The model under review builds one solid part; all positions refer to its coordinate system, in mm. Face numbers are marked on the shaded views. Give positions to 0.01 mm unless a question says otherwise; leave off trailing zeros. Order: outer loops, then holes, each group sorted by start corner. A loop starts at its lowest first (then second) coordinate and runs counter-clockwise, first axis right, second up. Notation, with made-up numbers: (-5, -39.75) - (16, -39.75) arc R27 cw to (16, -17.75) - close; hole circle Ø6 at (74, -15). An arc over 180 degrees is marked (long way). Use CSV: the item, a comma, the result in double quotes. Start each with the question number.
1. To check wall thickness, follow line 1 (Z direction, x = -6, y = 1.75); line 2 (Y direction, x = -7.25, z = -5.5); line 3 (X direction, y = 0.3, z = -4). State the ranges of each line that lie inside material, in increasing order. Write a range as [from, to].
2. Draft analysis for pull direction Z (two halves, no side actions). For the marked faces 1, 2, 3 and 4, state which applies: released by +Z, released by -Z, zero draft, split by the parting line, or undercut.
3. Take a section at D-D, the plane x = 7. State the section outline as (y, z) points.
4. Take a section at A-A, the plane x = 5. State the section outline as (y, z) points, then the cut area to 3 significant figures.
5. For pin 1 (2 mm diameter, centred on y = 3.5, z = -2.5, fed in from -X); pin 2 (1.5 mm diameter, centred on x = 1, y = 1.5, fed in from -Z); pin 3 (1 mm diameter, centred on y = 1.5, z = 6.5, fed in from +X), all flat-tipped, find the tip position at first contact; note any pin that passes through.
6. Take a section at B-B, the plane y = 0.6. State the section outline as (x, z) points, then the cut area to 3 significant figures.
7. Take a section at C-C, the plane x = -7.5. State the section outline as (y, z) points, then the cut area to 3 significant figures.
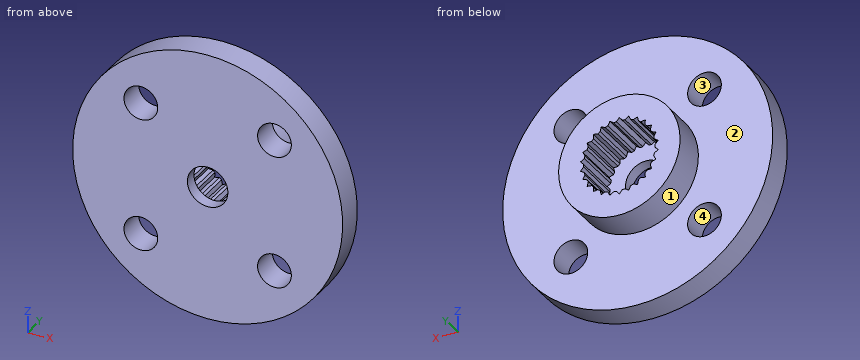
```python
from build123d import *

# Parameters (mm, degrees)
SKETCH_1_W              = 10
SKETCH_1_H              = 2
SKETCH_2_R              = 4.5
EXTRUDE_1_DEPTH         = 2.5
CUT_EXTRUDE_1_DEPTH     = 3.6
HOLE_WIZARD_3_0_3_1_D   = 3
HOLE_WIZARD_2_5_2_5_1_D = 2.5
CHAMFER_1_SIZE          = 0.140560122
CHAMFER_1_EDGE_2_SIZE   = 0.140560122
CHAMFER_1_EDGE_3_SIZE   = 0.140560122
CHAMFER_1_EDGE_4_SIZE   = 0.140560122
CHAMFER_1_EDGE_5_SIZE   = 0.140560122
CHAMFER_1_EDGE_6_SIZE   = 0.140560122
CHAMFER_1_EDGE_7_SIZE   = 0.140560122
CHAMFER_1_EDGE_8_SIZE   = 0.140560122
CHAMFER_1_EDGE_9_SIZE   = 0.140560122
CHAMFER_1_EDGE_10_SIZE  = 0.140560122
CHAMFER_1_EDGE_11_SIZE  = 0.140560122
CHAMFER_1_EDGE_12_SIZE  = 0.140560122
CHAMFER_1_EDGE_13_SIZE  = 0.140560122
CHAMFER_1_EDGE_14_SIZE  = 0.140560122
CHAMFER_1_EDGE_15_SIZE  = 0.140560122
CHAMFER_1_EDGE_16_SIZE  = 0.140560122
CHAMFER_1_EDGE_17_SIZE  = 0.140560122
CHAMFER_1_EDGE_18_SIZE  = 0.140560122
CHAMFER_1_EDGE_19_SIZE  = 0.140560122
CHAMFER_1_EDGE_20_SIZE  = 0.140560122
CHAMFER_1_EDGE_21_SIZE  = 0.140560122
CHAMFER_1_EDGE_22_SIZE  = 0.140560122
CHAMFER_1_EDGE_23_SIZE  = 0.140560122
CHAMFER_1_EDGE_24_SIZE  = 0.140560122
CHAMFER_1_EDGE_25_SIZE  = 0.140560122
CHAMFER_1_EDGE_26_SIZE  = 0.140560122


with BuildPart() as part:
    # Эскиз1 → Повернуть1 (revolve)
    with BuildSketch(Plane.XY, mode=Mode.PRIVATE) as revolve_1_sk:
        with Locations((5, 1)):
            Rectangle(SKETCH_1_W, SKETCH_1_H)
    revolve(revolve_1_sk.sketch.rotate(Axis((0, 2, 0), (0, -1, 0)), 270), axis=Axis((0, 2, 0), (0, -1, 0)))

    # Эскиз2 → Бобышка-Вытянуть1 (add)
    with BuildSketch(Plane(origin=(0, 2, 0), x_dir=(-1, 0, 0), z_dir=(0, 1, 0))):
        with Locations(Location((0, 0, 0), (0, 0, 90))):
            Circle(SKETCH_2_R)
    extrude(amount=EXTRUDE_1_DEPTH)

    # Эскиз3 → Вырез-Вытянуть1 (cut)
    with BuildSketch(Plane(origin=(0, 4.5, 0), x_dir=(-1, 0, 0), z_dir=(0, 1, 0))):
        Polygon((-2.711547104, 1.028354172), (-2.477853855, 0.610736123), (-2.878855735, 0.349556373), (-2.552010646, 0), (-2.878855735, -0.349556373), (-2.477853855, -0.610736123), (-2.711547104, -1.028354172), (-2.259693204, -1.185978483), (-2.386653211, -1.647387766), (-1.910207398, -1.692296084), (-1.923055709, -2.17068117), (-1.449707281, -2.100263587), (-1.347697199, -2.567822474), (-0.904955447, -2.386171406), (-0.694015426, -2.815731271), (-0.307610891, -2.533403615), (0, -2.9), (0.307610891, -2.533403615), (0.694015426, -2.815731271), (0.904955447, -2.386171406), (1.347697199, -2.567822474), (1.449707281, -2.100263587), (1.923055709, -2.17068117), (1.910207398, -1.692296084), (2.386653211, -1.647387766), (2.259693204, -1.185978483), (2.711547104, -1.028354172), (2.477853855, -0.610736123), (2.878855735, -0.349556373), (2.552010646, 0), (2.878855735, 0.349556373), (2.477853855, 0.610736123), (2.711547104, 1.028354172), (2.259693204, 1.185978483), (2.386653211, 1.647387766), (1.910207398, 1.692296084), (1.923055709, 2.17068117), (1.449707281, 2.100263587), (1.347697199, 2.567822474), (0.904955447, 2.386171406), (0.694015426, 2.815731271), (0.307610891, 2.533403615), (0, 2.9), (-0.307610891, 2.533403615), (-0.694015426, 2.815731271), (-0.904955447, 2.386171406), (-1.347697199, 2.567822474), (-1.449707281, 2.100263587), (-1.923055709, 2.17068117), (-1.910207398, 1.692296084), (-2.386653211, 1.647387766), (-2.259693204, 1.185978483), align=None)
    extrude(amount=-CUT_EXTRUDE_1_DEPTH, mode=Mode.SUBTRACT)

    # Диаметр отверстия Ø3.0 (3)1 (through all)
    with Locations(Plane(origin=(0, 0.9, 0), x_dir=(1, 0, 0), z_dir=(0, 1, 0))):
        with Locations((0, 0)):
            Hole(HOLE_WIZARD_3_0_3_1_D / 2)

    # Диаметр отверстия Ø2.5 (2.5)1 (through all)
    with Locations(Plane(origin=(0, 2, 0), x_dir=(1, 0, 0), z_dir=(0, 1, 0))):
        with Locations((-4.949747468, 4.949747468), (4.949747468, 4.949747468), (4.949747468, -4.949747468), (-4.949747468, -4.949747468)):
            Hole(HOLE_WIZARD_2_5_2_5_1_D / 2)

    # Фаска1
    chamfer_1_edges = [part.edges().sort_by_distance(p)[0] for p in [
        (2.259693204, 2.7, 1.185978483),
    ]]
    chamfer(chamfer_1_edges, length=CHAMFER_1_SIZE)

    # Фаска1 edge 2
    chamfer_1_edge_2_edges = [part.edges().sort_by_distance(p)[0] for p in [
        (1.910207398, 2.7, 1.692296084),
    ]]
    chamfer(chamfer_1_edge_2_edges, length=CHAMFER_1_EDGE_2_SIZE)

    # Фаска1 edge 3
    chamfer_1_edge_3_edges = [part.edges().sort_by_distance(p)[0] for p in [
        (1.449707281, 2.7, 2.100263587),
    ]]
    chamfer(chamfer_1_edge_3_edges, length=CHAMFER_1_EDGE_3_SIZE)

    # Фаска1 edge 4
    chamfer_1_edge_4_edges = [part.edges().sort_by_distance(p)[0] for p in [
        (0.904955447, 2.7, 2.386171406),
    ]]
    chamfer(chamfer_1_edge_4_edges, length=CHAMFER_1_EDGE_4_SIZE)

    # Фаска1 edge 5
    chamfer_1_edge_5_edges = [part.edges().sort_by_distance(p)[0] for p in [
        (0.307610891, 2.7, 2.533403615),
    ]]
    chamfer(chamfer_1_edge_5_edges, length=CHAMFER_1_EDGE_5_SIZE)

    # Фаска1 edge 6
    chamfer_1_edge_6_edges = [part.edges().sort_by_distance(p)[0] for p in [
        (-0.307610891, 2.7, 2.533403615),
    ]]
    chamfer(chamfer_1_edge_6_edges, length=CHAMFER_1_EDGE_6_SIZE)

    # Фаска1 edge 7
    chamfer_1_edge_7_edges = [part.edges().sort_by_distance(p)[0] for p in [
        (-0.904955447, 2.7, 2.386171406),
    ]]
    chamfer(chamfer_1_edge_7_edges, length=CHAMFER_1_EDGE_7_SIZE)

    # Фаска1 edge 8
    chamfer_1_edge_8_edges = [part.edges().sort_by_distance(p)[0] for p in [
        (-1.449707281, 2.7, 2.100263587),
    ]]
    chamfer(chamfer_1_edge_8_edges, length=CHAMFER_1_EDGE_8_SIZE)

    # Фаска1 edge 9
    chamfer_1_edge_9_edges = [part.edges().sort_by_distance(p)[0] for p in [
        (-1.910207398, 2.7, 1.692296084),
    ]]
    chamfer(chamfer_1_edge_9_edges, length=CHAMFER_1_EDGE_9_SIZE)

    # Фаска1 edge 10
    chamfer_1_edge_10_edges = [part.edges().sort_by_distance(p)[0] for p in [
        (-2.259693204, 2.7, 1.185978483),
    ]]
    chamfer(chamfer_1_edge_10_edges, length=CHAMFER_1_EDGE_10_SIZE)

    # Фаска1 edge 11
    chamfer_1_edge_11_edges = [part.edges().sort_by_distance(p)[0] for p in [
        (-2.477853855, 2.7, 0.610736123),
    ]]
    chamfer(chamfer_1_edge_11_edges, length=CHAMFER_1_EDGE_11_SIZE)

    # Фаска1 edge 12
    chamfer_1_edge_12_edges = [part.edges().sort_by_distance(p)[0] for p in [
        (-2.552010646, 2.7, 0),
    ]]
    chamfer(chamfer_1_edge_12_edges, length=CHAMFER_1_EDGE_12_SIZE)

    # Фаска1 edge 13
    chamfer_1_edge_13_edges = [part.edges().sort_by_distance(p)[0] for p in [
        (-2.477853855, 2.7, -0.610736123),
    ]]
    chamfer(chamfer_1_edge_13_edges, length=CHAMFER_1_EDGE_13_SIZE)

    # Фаска1 edge 14
    chamfer_1_edge_14_edges = [part.edges().sort_by_distance(p)[0] for p in [
        (-2.259693204, 2.7, -1.185978483),
    ]]
    chamfer(chamfer_1_edge_14_edges, length=CHAMFER_1_EDGE_14_SIZE)

    # Фаска1 edge 15
    chamfer_1_edge_15_edges = [part.edges().sort_by_distance(p)[0] for p in [
        (-1.910207398, 2.7, -1.692296084),
    ]]
    chamfer(chamfer_1_edge_15_edges, length=CHAMFER_1_EDGE_15_SIZE)

    # Фаска1 edge 16
    chamfer_1_edge_16_edges = [part.edges().sort_by_distance(p)[0] for p in [
        (-1.449707281, 2.7, -2.100263587),
    ]]
    chamfer(chamfer_1_edge_16_edges, length=CHAMFER_1_EDGE_16_SIZE)

    # Фаска1 edge 17
    chamfer_1_edge_17_edges = [part.edges().sort_by_distance(p)[0] for p in [
        (-0.904955447, 2.7, -2.386171406),
    ]]
    chamfer(chamfer_1_edge_17_edges, length=CHAMFER_1_EDGE_17_SIZE)

    # Фаска1 edge 18
    chamfer_1_edge_18_edges = [part.edges().sort_by_distance(p)[0] for p in [
        (-0.307610891, 2.7, -2.533403615),
    ]]
    chamfer(chamfer_1_edge_18_edges, length=CHAMFER_1_EDGE_18_SIZE)

    # Фаска1 edge 19
    chamfer_1_edge_19_edges = [part.edges().sort_by_distance(p)[0] for p in [
        (0.307610891, 2.7, -2.533403615),
    ]]
    chamfer(chamfer_1_edge_19_edges, length=CHAMFER_1_EDGE_19_SIZE)

    # Фаска1 edge 20
    chamfer_1_edge_20_edges = [part.edges().sort_by_distance(p)[0] for p in [
        (0.904955447, 2.7, -2.386171406),
    ]]
    chamfer(chamfer_1_edge_20_edges, length=CHAMFER_1_EDGE_20_SIZE)

    # Фаска1 edge 21
    chamfer_1_edge_21_edges = [part.edges().sort_by_distance(p)[0] for p in [
        (1.449707281, 2.7, -2.100263587),
    ]]
    chamfer(chamfer_1_edge_21_edges, length=CHAMFER_1_EDGE_21_SIZE)

    # Фаска1 edge 22
    chamfer_1_edge_22_edges = [part.edges().sort_by_distance(p)[0] for p in [
        (1.910207398, 2.7, -1.692296084),
    ]]
    chamfer(chamfer_1_edge_22_edges, length=CHAMFER_1_EDGE_22_SIZE)

    # Фаска1 edge 23
    chamfer_1_edge_23_edges = [part.edges().sort_by_distance(p)[0] for p in [
        (2.259693204, 2.7, -1.185978483),
    ]]
    chamfer(chamfer_1_edge_23_edges, length=CHAMFER_1_EDGE_23_SIZE)

    # Фаска1 edge 24
    chamfer_1_edge_24_edges = [part.edges().sort_by_distance(p)[0] for p in [
        (2.477853855, 2.7, -0.610736123),
    ]]
    chamfer(chamfer_1_edge_24_edges, length=CHAMFER_1_EDGE_24_SIZE)

    # Фаска1 edge 25
    chamfer_1_edge_25_edges = [part.edges().sort_by_distance(p)[0] for p in [
        (2.552010646, 2.7, 0),
    ]]
    chamfer(chamfer_1_edge_25_edges, length=CHAMFER_1_EDGE_25_SIZE)

    # Фаска1 edge 26
    chamfer_1_edge_26_edges = [part.edges().sort_by_distance(p)[0] for p in [
        (2.477853855, 2.7, 0.610736123),
    ]]
    chamfer(chamfer_1_edge_26_edges, length=CHAMFER_1_EDGE_26_SIZE)


solid = part.part
```
Determined:
1,line 1,"z = [-8, -5.63], [-4.27, 4.27], [5.63, 8]"
1,line 2,"y = [0, 2]"
1,line 3,"x = [-9.17, -5.76], [-4.14, 4.14], [5.76, 9.17]"
2,face 1,"split by the parting line"
2,face 2,"zero draft"
2,face 3,"undercut"
2,face 4,"undercut"
3,outline,"(0, -7.14) - (2, -7.14) - (2, 7.14) - (0, 7.14) - close"
4,outline,"(0, -8.66) - (2, -8.66) - (2, -6.2) - (0, -6.2) - close; (0, -3.7) - (2, -3.7) - (2, 3.7) - (0, 3.7) - close; (0, 6.2) - (2, 6.2) - (2, 8.66) - (0, 8.66) - close"
4,area,"24.6 mm²"
5,pin 1,"stops at x = -4.24"
5,pin 2,"stops at z = -10"
5,pin 3,"stops at x = 8"
6,outline,"circle Ø20 at (0, 0); hole circle Ø2.5 at (-4.95, -4.95); hole circle Ø2.5 at (-4.95, 4.95); hole circle Ø3 at (0, 0); hole circle Ø2.5 at (4.95, -4.95); hole circle Ø2.5 at (4.95, 4.95)"
6,area,"287 mm²"
7,outline,"(0, -6.61) - (2, -6.61) - (2, 6.61) - (0, 6.61) - close"
7,area,"26.5 mm²"
